from build123d import *

# Parameters (mm, degrees)
SALIENTE_EXTRUIR2_DEPTH    = 40
CROQUIS2_R                 = 12.5
SALIENTE_EXTRUIR3_DEPTH    = 4.5
CROQUIS3_R                 = 10
SALIENTE_EXTRUIR4_DEPTH    = 21.5
CORTAR_EXTRUIR1_DEPTH      = 21.5
CORTAR_EXTRUIR1_DEPTH_BACK = 21.5
CROQUIS4_R                 = 3.5
CROQUIS5_R                 = 25
SALIENTE_EXTRUIR5_DEPTH    = 30
CROQUIS6_W                 = 110
CROQUIS6_H                 = 50
SALIENTE_EXTRUIR6_DEPTH    = 60
CROQUIS10_W                = 45
CROQUIS10_H                = 50
SALIENTE_EXTRUIR7_DEPTH    = 30
CROQUIS12_W                = 50
CROQUIS12_H                = 55
SALIENTE_EXTRUIR8_DEPTH    = 20
CROQUIS13_R                = 20
SALIENTE_EXTRUIR9_DEPTH    = 70
CROQUIS14_W                = 10
CROQUIS14_H                = 60
SALIENTE_EXTRUIR10_DEPTH   = 90
CORTAR_EXTRUIR4_START      = -100
CORTAR_EXTRUIR4_OUTLINE_R  = 6
CORTAR_EXTRUIR4_DEPTH      = 101
CROQUIS16_R                = 25
SALIENTE_EXTRUIR11_DEPTH   = 800


with BuildPart() as part:
    # Croquis1 → Saliente-Extruir2 (new body)
    with BuildSketch(Plane(origin=(0, 0, 0), x_dir=(1, 0, 0), z_dir=(0, 1, 0))):
        with BuildLine():
            Line((-50, 19.52562419), (-50, -60))
            Line((-50, -60), (50, -60))
            Line((50, -60), (50, 19.52562419))
            ThreePointArc((50, 19.52562419), (0, 60), (-50, 19.52562419))
        make_face()
    extrude(amount=SALIENTE_EXTRUIR2_DEPTH)

    # Croquis2 → Saliente-Extruir3 (add)
    with BuildSketch(Plane(origin=(0, 40, 0), x_dir=(1, 0, 0), z_dir=(0, 1, 0))):
        with Locations(Location((0, 15, 0), (0, 0, 270))):
            Circle(CROQUIS2_R)
    extrude(amount=SALIENTE_EXTRUIR3_DEPTH)

    # Croquis3 → Saliente-Extruir4 (add)
    with BuildSketch(Plane(origin=(0, 44.5, 0), x_dir=(1, 0, 0), z_dir=(0, 1, 0))):
        with Locations(Location((0, 15, 0), (0, 0, 270))):
            Circle(CROQUIS3_R)
    extrude(amount=SALIENTE_EXTRUIR4_DEPTH)

    # Croquis4 → Cortar-Extruir1 (cut, two sides: drawn at the far end of the back side and taken through both)
    with BuildSketch(Plane(origin=(0, 0, 0), x_dir=(0, 0, -1), z_dir=(1, 0, 0)).offset(-CORTAR_EXTRUIR1_DEPTH_BACK)):
        with Locations(Location((15, 54.5, 0), (0, 0, 180))):
            Circle(CROQUIS4_R)
    extrude(amount=CORTAR_EXTRUIR1_DEPTH + CORTAR_EXTRUIR1_DEPTH_BACK, mode=Mode.SUBTRACT)

    # Chafl_n1: read off the stored shape, not the designer's step
    # Chafl_n1 outline → Chafl_n1 (revolve, cut)
    with BuildSketch(Plane.XY.offset(-15)):
        Polygon((10, 66), (9, 66), (10, 65), align=None)
    revolve(axis=Axis((0, 0, -15), (0, 1, 0)), mode=Mode.SUBTRACT)

    # Croquis5 → Saliente-Extruir5 (add)
    with BuildSketch(Plane.ZY.offset(50)):
        with Locations(Location((30, 20, 0), (0, 0, 126.869897646))):
            Circle(CROQUIS5_R)
    extrude(amount=SALIENTE_EXTRUIR5_DEPTH)

    # Croquis6 → Saliente-Extruir6 (add)
    with BuildSketch(Plane.ZY.offset(80)):
        with Locations((60.2509382, 21.110140405)):
            Rectangle(CROQUIS6_W, CROQUIS6_H)
    extrude(amount=SALIENTE_EXTRUIR6_DEPTH)

    # Croquis10 → Saliente-Extruir7 (add)
    with BuildSketch(Plane(origin=(-80, 0, 0), x_dir=(0, 0, -1), z_dir=(1, 0, 0))):
        with Locations((-92.7509382, 21.110140405)):
            Rectangle(CROQUIS10_W, CROQUIS10_H)
    extrude(amount=SALIENTE_EXTRUIR7_DEPTH)

    # Croquis12 → Saliente-Extruir8 (add)
    with BuildSketch(Plane(origin=(-50, 0, 0), x_dir=(0, 0, -1), z_dir=(1, 0, 0))):
        with Locations((-92.7509382, 21.110140405)):
            Rectangle(CROQUIS12_W, CROQUIS12_H)
    extrude(amount=SALIENTE_EXTRUIR8_DEPTH)

    # Croquis13 → Saliente-Extruir9 (add)
    with BuildSketch(Plane(origin=(-30, 0, 0), x_dir=(0, 0, -1), z_dir=(1, 0, 0))):
        with Locations((-92.7509382, 21.110140405)):
            Circle(CROQUIS13_R)
    extrude(amount=SALIENTE_EXTRUIR9_DEPTH)

    # Croquis14 → Saliente-Extruir10 (add)
    with BuildSketch(Plane.XZ):
        with Locations((-45, 10.47437581)):
            Rectangle(CROQUIS14_W, CROQUIS14_H)
    saliente_extruir10 = extrude(amount=SALIENTE_EXTRUIR10_DEPTH)

    # Simetr_a1: Saliente-Extruir10 across plane
    add(saliente_extruir10.mirror(Plane(origin=(0, 0, 0), x_dir=(0, 0, 1), z_dir=(1, 0, 0))))

    # Cortar-Extruir4: read off the stored shape, not the designer's step
    # Cortar-Extruir4 outline → Cortar-Extruir4 (cut)
    with BuildSketch(Plane.ZY.offset(50).offset(CORTAR_EXTRUIR4_START)):
        with BuildLine():
            ThreePointArc((40.47437581, -60), (31.687579246, -81.213203436), (10.47437581, -90))
            Line((10.47437581, -90), (40.47437581, -90))
            Line((40.47437581, -90), (40.47437581, -60))
        make_face()
        with BuildLine():
            ThreePointArc((10.47437581, -90), (-10.738827626, -81.213203436), (-19.52562419, -60))
            Line((-19.52562419, -60), (-19.52562419, -90))
            Line((-19.52562419, -90), (10.47437581, -90))
        make_face()
        with Locations((10.47437581, -60)):
            Circle(CORTAR_EXTRUIR4_OUTLINE_R)
    extrude(amount=CORTAR_EXTRUIR4_DEPTH, mode=Mode.SUBTRACT)

    # Croquis16 → Saliente-Extruir11 (add)
    with BuildSketch(Plane(origin=(0, 0, 0), x_dir=(-1, 0, 0), z_dir=(0, -1, 0))):
        with Locations(Location((0, 0, 0), (0, 0, 90))):
            Circle(CROQUIS16_R)
    extrude(amount=SALIENTE_EXTRUIR11_DEPTH)


solid = part.part
CAD build for the part. Positions are in the model's coordinates, mm. A direction names the side the tool comes from. Coordinates: 2 decimals unless noted, no trailing zeros. Loops run counter-clockwise (first coordinate to the right, second up) from the corner with the lowest first, then second, coordinate; pieces in that order, holes last. Notation, with made-up numbers: (86.5, 7.25) - (106.5, 7.25) arc R22 ccw to (106.5, 21.25) - close; hole circle Ø1 at (-16, 1). An arc over 180 degrees is marked (long way). Use one line per item in the form item = value. Start each with the question number.
1) Band-saw the part on D-D (z = -40.5). Give the cut face in (x, y).
2) Drill centre lines: L1, parallel to Z at x = -45, y = -60; L2, parallel to Z at x = -0.75, y = 54.5; L3, parallel to Y at x = 0.25, z = -15. Where is each one in solid material? Low to high. Write a range as from..to.
3) Band-saw the part on B-B (x = 0). Give the cut face in (y, z), and give its area (3 significant figures).
4) Flat gauge pins, fed straight in: pin 1 (8 mm diameter, centred on x = -47, y = -16.5, fed in from -Z); pin 2 (8 mm diameter, centred on x = 43, y = -21.5, fed in from +Z); pin 3 (8 mm diameter, centred on y = 54.5, z = -15, fed in from +X). Where does each tip first touch, or does it go through?
5) Band-saw the part on C-C (y = -433). Give the cut face in (x, z).
6) Tool access for faces 4 (the face through (-40, -44, 10)), 5 (the face through (-1, 20, 60)), 6 (the face through (10.2, 44.5, -15.1)), 7 (the face through (-30, 34, 76)): list every direction of +Z, -Z, +X, -X, +Y, -Y with a clear straight run to the whole face (end or side of a thin tool).
7) Two-plate mould, pull along Z, no slides. Class faces 1 (the face through (-106, 46.11, 61)), 2 (the face through (-40, 21, 67.751)), 3 (the face through (3, 54.61, -5.46)): +Z half, -Z half, draft (parallel to the pull), parting line (faces both ways), or undercut.
8) Band-saw the part on A-A (y = -26). Give the cut face in (x, z).
Check values:
q1.outline = (-40.17, 0) - (40.17, 0) - (40.17, 40) - (-40.17, 40) - close
q2.L1 = -19.53..4.47, 16.47..40.47
q2.L2 = -24.97..-18.5, -11.5..-5.03
q2.L3 = -800..51, 58..66
q3.outline = (-800, -25) - (0, -25) - (0, -60) - (40, -60) - (40, -27.5) - (44.5, -27.5) - (44.5, -25) - (65, -25) - (66, -24) - (66, -6) - (65, -5) - (44.5, -5) - (44.5, -2.5) - (40, -2.5) - (40, 60) - (0, 60) - (0, 25) - (-800, 25) - close; circle Ø40 at (21.11, 92.75); hole circle Ø7 at (54.5, -15)
q3.area = 46,600 mm2
q4.pin_1 = -19.53
q4.pin_2 = 40.47
q4.pin_3 = 10
q5.outline = circle Ø50 at (0, 0)
q6.face_4 = -Z, -Y
q6.face_5 = +X, +Y, -Y
q6.face_6 = +Y
q6.face_7 = +X
q7.face_1 = draft
q7.face_2 = undercut
q7.face_3 = parting line
q8.outline = (-50, -19.53) - (-40, -19.53) - (-40, 40.47) - (-50, 40.47) - close; circle Ø50 at (0, 0); (40, -19.53) - (50, -19.53) - (50, 40.47) - (40, 40.47) - close
